Input: dimensioned drawing with shaded views. Units: mm. Origin: part minimum x, y, z. Coordinates: 2 decimals unless noted, no trailing zeros. Loops run counter-clockwise (first coordinate to the right, second up) from the corner with the lowest first, then second, coordinate; pieces in that order, holes last.
(1) Line query: L1, parallel to Z at x = 10.25, y = 50; L2, parallel to Y at x = 15.25, z = 33; L3, parallel to Y at x = 4, z = 74. Output: solid intervals per line, ascending.
(2) Section C-C, the plane x = 9. Return loops of the section in (y, z).
(3) Mould query, pull axis Y, two halves, no side actions, for the marked faces 1, 2, 3 and 4. Classes: released by +Y, released by -Y, zero draft, split by the parting line, or undercut.
(4) Section B-B, the plane y = 55. Return loops of the section in (x, z), then the cut area to 3 significant figures.
(5) Section A-A, the plane z = 50. Return loops of the section in (x, y).
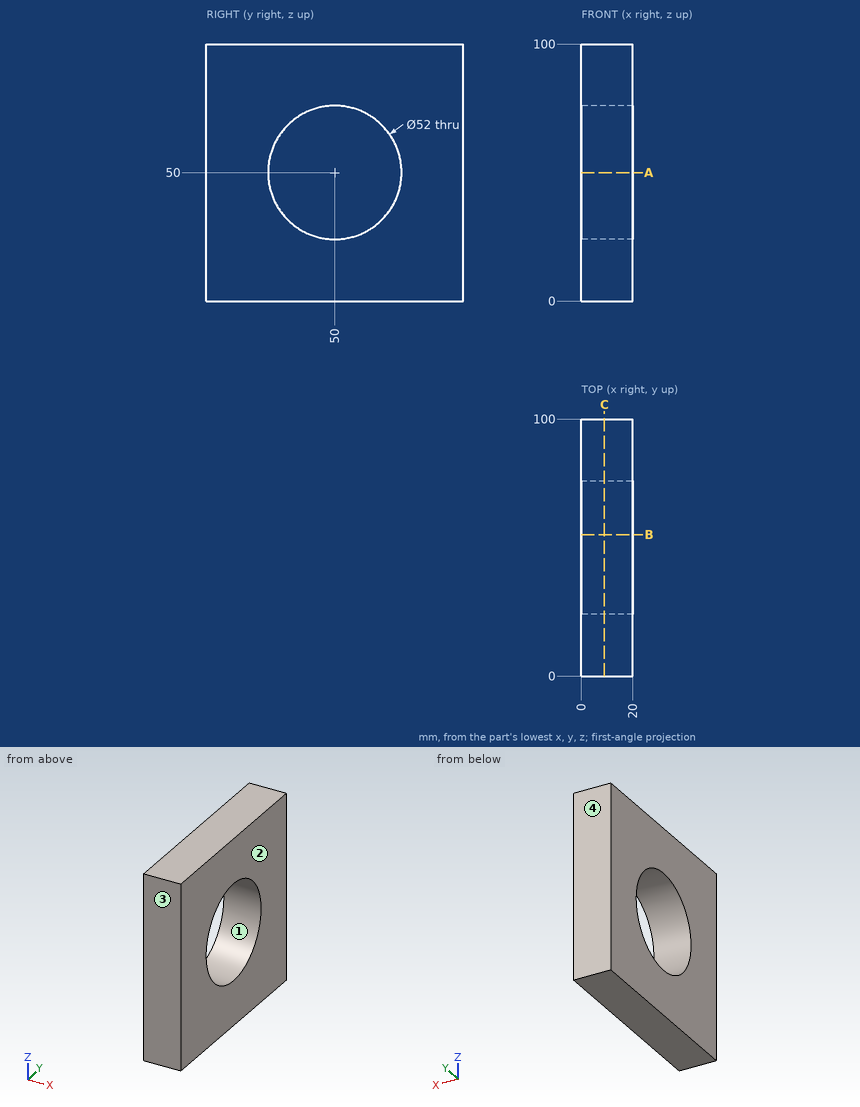
Report:
1. L1: z = 0 to 24, 76 to 100
1. L2: y = 0 to 30.33, 69.67 to 100
1. L3: y = 0 to 40, 60 to 100
2. outline: (0, 0) - (100, 0) - (100, 100) - (0, 100) - close; hole circle Ø52 at (50, 50)
3. face 1: undercut
3. face 2: zero draft
3. face 3: released by -Y
3. face 4: released by +Y
4. outline: (0, 0) - (20, 0) - (20, 24.49) - (0, 24.49) - close; (0, 75.51) - (20, 75.51) - (20, 100) - (0, 100) - close
4. area: 979 mm2
5. outline: (0, 0) - (20, 0) - (20, 24) - (0, 24) - close; (0, 76) - (20, 76) - (20, 100) - (0, 100) - close
